```python
from build123d import *

# Parameters (mm, degrees)
CUT_EXTRUDE1_DEPTH       = 19.66511184
FILLET2_R                = 0.508
CIRPATTERN1_COUNT        = 18
FILLET2_OF_CIRPATTERN1_R = 0.508


with BuildPart() as part:
    # Sketch1 → Revolve1 (revolve)
    with BuildSketch(Plane.XY, mode=Mode.PRIVATE) as revolve1_sk:
        Polygon((5.08, 5.842), (3.048, 5.842), (3.048, 10.16), (5.08, 10.16), (5.08, 12.7), (-5.08, 12.7), (-5.08, 10.16), (-3.048, 10.16), (-3.048, 5.842), (-5.08, 5.842), (-5.08, 3.302), (5.08, 3.302), align=None)
    revolve(revolve1_sk.sketch.rotate(Axis((0, 0, 0), (1, 0, 0)), 90), axis=Axis((0, 0, 0), (1, 0, 0)))

    # Sketch2 → Cut-Extrude1 (cut, symmetric)
    with BuildSketch(Plane(origin=(0, 0, 0), x_dir=(0, 0, -1), z_dir=(1, 0, 0))):
        Polygon((0.635, 11.291535111), (1.991281675, 12.906814359), (-1.991281675, 12.906814359), (-0.635, 11.291535111), align=None)
    cut_extrude1 = extrude(amount=CUT_EXTRUDE1_DEPTH, both=True, mode=Mode.SUBTRACT)

    # Fillet2
    fillet2_edges = [part.edges().sort_by_distance(p)[0] for p in [
        (0, 12.583064675, 1.719442756),
        (0, 12.583064675, -1.719442756),
    ]]
    fillet(fillet2_edges, radius=FILLET2_R)

    # CirPattern1: Cut-Extrude1 ×18 about axis
    cirpattern1_axis = Axis((0, 0, 0), (1, 0, 0))
    for i in range(1, CIRPATTERN1_COUNT):
        add(cut_extrude1.rotate(cirpattern1_axis, i * 360 / CIRPATTERN1_COUNT), mode=Mode.SUBTRACT)

    # Fillet2 of CirPattern1
    fillet2_of_cirpattern1_edges = [part.edges().sort_by_distance(p)[0] for p in [
        (0, 11.236128964, 5.919409254),
        (0, 12.41229708, 2.687913913),
        (0, 8.533950272, 9.405407634),
        (0, 10.744423271, 6.771068496),
        (0, 4.80245123, 11.756975044),
        (0, 7.780613445, 10.037532288),
        (0, 0.491705693, 12.69047775),
        (0, 3.878346808, 12.093321547),
        (0, -3.878346808, 12.093321547),
        (0, -0.491705693, 12.69047775),
        (0, -7.780613445, 10.037532288),
        (0, -4.80245123, 11.756975044),
        (0, -10.744423271, 6.771068496),
        (0, -8.533950272, 9.405407634),
        (0, -12.41229708, 2.687913913),
        (0, -11.236128964, 5.919409254),
        (0, -12.583064675, -1.719442756),
        (0, -12.583064675, 1.719442756),
        (0, -11.236128964, -5.919409254),
        (0, -12.41229708, -2.687913913),
        (0, -8.533950272, -9.405407634),
        (0, -10.744423271, -6.771068496),
        (0, -4.80245123, -11.756975044),
        (0, -7.780613445, -10.037532288),
        (0, -0.491705693, -12.69047775),
        (0, -3.878346808, -12.093321547),
        (0, 3.878346808, -12.093321547),
        (0, 0.491705693, -12.69047775),
        (0, 7.780613445, -10.037532288),
        (0, 4.80245123, -11.756975044),
        (0, 10.744423271, -6.771068496),
        (0, 8.533950272, -9.405407634),
        (0, 12.41229708, -2.687913913),
        (0, 11.236128964, -5.919409254),
    ]]
    fillet(fillet2_of_cirpattern1_edges, radius=FILLET2_OF_CIRPATTERN1_R)


solid = part.part
```
Check sheet for the modelled part. Datum: model origin and axes. Units: mm. A direction names the side the tool comes from. Round coordinates to 2 decimals unless told otherwise and drop trailing zeros. Write each loop counter-clockwise with the first axis right and the second up, starting at its lowest first coordinate (ties: lowest second). Pieces come first, ordered by that corner, then holes. Notation, with made-up numbers: (-3.75, 3) -> (10.25, 3) arc R27 ccw to (10.25, 37) -> close; hole circle Ø4 at (51, 88). An arc over 180 degrees is marked (long way). One line per question, with ' | ' between items. Start each with the question number.
1. Depth check by flat-ended pin: pin 1 (1 mm diameter, centred on x = -0.5, y = -4.5, fed in from -Z); pin 2 (1.5 mm diameter, centred on x = -0.5, z = 7, fed in from +Y); pin 3 (0.6 mm diameter, centred on x = 0, z = 0.5, fed in from -Y). Enter the tip coordinate at first touch or a pass-through.
2. Set-up check for faces 1 (the face through (-4.05, -10.074, -1.323)), 2 (the face through (0.07, 11.82, -1.08)), 3 (the face through (0.071, -0.98, -11.846)), 4 (the face through (0.07, -11.5, 3.02)): record each of +Z, -Z, +X, -X, +Y, -Y from which the full face is reachable in a straight line by a thin tool's end or side.
3. Sectioned sample at C-C, the plane z = 10.5. Record the cut outline in (x, y), then the cut area to 3 significant figures.
4. Sectioned sample at A-A, the plane z = 0. Record the cut outline in (x, y), then the cut area to 3 significant figures.
5. Scan lines: line 1 along Y through (x, z) = (4.45, 0); line 2 along Z through (x, y) = (-4.25, 3); line 3 along Y through (x, z) = (-3, 0.5). Record each from-to range of solid material in increasing order. Write a range as from..to.
6. Sectioned sample at B-B, the plane x = -4.5. Count the separate pieces of the cut face and the enclosed holes in it, then the cut area to 3 significant figures.
7. Release check for a two-part mould opening along Y. For faces 5 (the face through (4.078, -10.074, -1.323)), 6 (the face through (0.071, -10.749, -5.075)), 7 (the face through (4, 3.6, -4.6)), 8 (the face through (0.071, 11.836, 1.092)) record: +Y half, -Y half, draft (parallel to the pull), parting line (faces both ways), or undercut.
Taken from the geometry:
1) pin 1: stops at z = -12.03 | pin 2: stops at y = 11.06 | pin 3: stops at y = -11.49
2) face 1: -X | face 2: +X, -X, +Y | face 3: -Z, +X, -X | face 4: +X, -X, -Y
3) outline: (-5.08, -5.02) -> (5.08, -5.02) -> (5.08, 5.02) -> (-5.08, 5.02) -> close | area: 102 mm^2
4) outline: (-5.08, -11.29) -> (5.08, -11.29) -> (5.08, -10.16) -> (3.05, -10.16) -> (3.05, -5.84) -> (5.08, -5.84) -> (5.08, -3.3) -> (-5.08, -3.3) -> (-5.08, -5.84) -> (-3.05, -5.84) -> (-3.05, -10.16) -> (-5.08, -10.16) -> close; (-5.08, 3.3) -> (5.08, 3.3) -> (5.08, 5.84) -> (3.05, 5.84) -> (3.05, 10.16) -> (5.08, 10.16) -> (5.08, 11.29) -> (-5.08, 11.29) -> (-5.08, 10.16) -> (-3.05, 10.16) -> (-3.05, 5.84) -> (-5.08, 5.84) -> close | area: 127 mm^2
5) line 1: y = -11.29..-10.16, -5.84..-3.3, 3.3..5.84, 10.16..11.29 | line 2: z = -11.36..-9.71, -5.01..-1.38, 1.38..5.01, 9.71..11.36 | line 3: y = -11.29..-3.26, 3.26..11.29
6) separate pieces: 2 | enclosed holes: 2 | area: 195 mm^2
7) face 5: undercut | face 6: -Y half | face 7: undercut | face 8: +Y half
